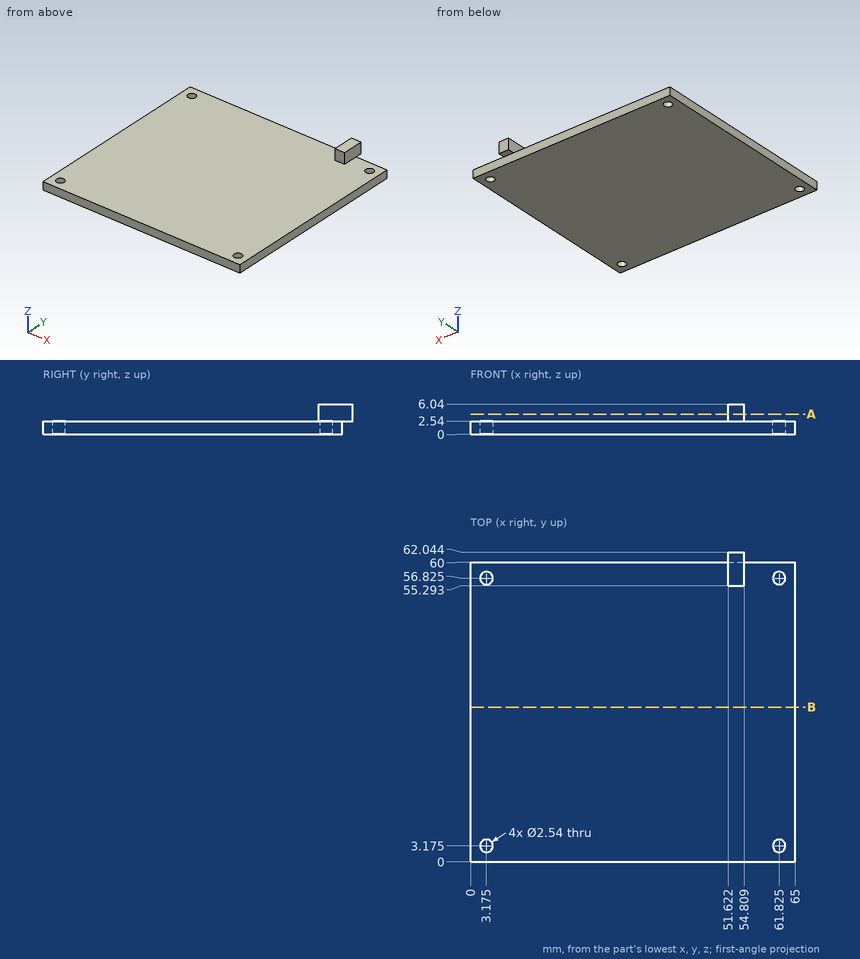
Here's the drawing with two shaded views (mm, measured from the low corner). I have some questions. Coordinates: 2 decimals unless noted, no trailing zeros. Loops run counter-clockwise (first coordinate to the right, second up) from the corner with the lowest first, then second, coordinate; pieces in that order, holes last. Notation, with made-up numbers: (78, 88.25) -> (95, 88.25) arc R35 ccw to (95, 120.25) -> close; hole circle Ø9 at (76.25, 51). An arc over 180 degrees is marked (long way). Put each result on its own line as item: value. Start each with the question number.
Q1. I want a section at B-B (y = 31). Write out the boundary of the cut face in (x, z), plus the area to 3 significant figures.
Q2. I want a section at A-A (z = 4). Write out the boundary of the cut face in (x, y) (1 decimal), plus the area to 3 significant figures.
Q3. I'm going to push flat-ended pins straight in: P1, Ø2, axis at x = 61.825, y = 56.825, coming from the -Z side; P2, Ø2, axis at x = 35.5, z = 1, coming from the +Y side; P3, Ø3, axis at x = 50, y = 22, coming from the +Z side; P4, Ø3, axis at y = 59.5, z = 4.5, coming from the +X side. Where does each tip first touch, or does it pass through?
Q4. If I drill on line 1 (Y direction, x = 62, z = 2.25); line 2 (Z direction, x = 33.5, y = 25.5); line 3 (Y direction, x = 21.5, z = 2.25), over which ranges is the centre line in solid material (lowest first)? Write a range as [from, to].
Taken from the geometry:
1. outline: (0, 0) -> (65, 0) -> (65, 2.54) -> (0, 2.54) -> close
1. area: 165 mm2
2. outline: (51.6, 55.3) -> (54.8, 55.3) -> (54.8, 62) -> (51.6, 62) -> close
2. area: 21.5 mm2
3. P1: passes through
3. P2: stops at y = 60
3. P3: stops at z = 2.54
3. P4: stops at x = 54.81
4. line 1: y = [0, 1.92], [4.43, 55.57], [58.08, 60]
4. line 2: z = [0, 2.54]
4. line 3: y = [0, 60]
